```python
from build123d import *

# Parameters (mm, degrees)
SKETCH_1_R          = 21.15
SKETCH_1_R_2        = 1.5
EXTRUDE_1_DEPTH     = 4
SKETCH_2_W          = 6
SKETCH_2_H          = 5
CUT_EXTRUDE_1_DEPTH = 98.49871794


with BuildPart() as part:
    # 草图1 → 凸台-拉伸1 (new body)
    with BuildSketch(Plane.XY):
        with BuildLine():
            Line((-29, 6), (29, 6))
            Line((29, 6), (29, -64))
            ThreePointArc((29, -64), (0, -93), (-29, -64))
            Line((-29, -64), (-29, 6))
        make_face()
        with Locations((0, -64)):
            Circle(SKETCH_1_R, mode=Mode.SUBTRACT)
        with Locations((-17.5, 3)):
            Circle(SKETCH_1_R_2, mode=Mode.SUBTRACT)
        with Locations((17.5, 3)):
            Circle(SKETCH_1_R_2, mode=Mode.SUBTRACT)
        with Locations((18.561553006, -82.561553006)):
            Circle(SKETCH_1_R_2, mode=Mode.SUBTRACT)
        with Locations((-18.561553006, -82.561553006)):
            Circle(SKETCH_1_R_2, mode=Mode.SUBTRACT)
        with Locations((-18.561553006, -45.438446994)):
            Circle(SKETCH_1_R_2, mode=Mode.SUBTRACT)
        with Locations((18.561553006, -45.438446994)):
            Circle(SKETCH_1_R_2, mode=Mode.SUBTRACT)
        with Locations((-17.5, -3)):
            Circle(SKETCH_1_R_2, mode=Mode.SUBTRACT)
        with Locations((17.5, -3)):
            Circle(SKETCH_1_R_2, mode=Mode.SUBTRACT)
    extrude(amount=EXTRUDE_1_DEPTH)

    # 草图2 → 切除-拉伸1 (cut, through all)
    with BuildSketch(Plane.XY.offset(4)):
        with Locations((0, 3.5)):
            Rectangle(SKETCH_2_W, SKETCH_2_H)
    extrude(amount=-CUT_EXTRUDE_1_DEPTH, mode=Mode.SUBTRACT)


solid = part.part
```
Geometry: final body of the model. Coordinates: model frame, mm. A direction names the side the tool comes from. Round coordinates to 2 decimals unless told otherwise and drop trailing zeros. Write each loop counter-clockwise with the first axis right and the second up, starting at its lowest first coordinate (ties: lowest second). Pieces come first, ordered by that corner, then holes. Notation, with made-up numbers: M 24.5,39 L 33.5,39 A19 ccw 33.5,51 Z; hole C -9.75,35.5 d10. An arc over 180 degrees is marked long. Answer in a Markdown table with one row per item. Add a question column.
(1) Contact query for flat-ended pins moving along their axis: pin 1 (3.5 mm diameter, centred on x = -17.5, y = 3, fed in from +Z); pin 2 (2.5 mm diameter, centred on x = -18.56, y = -82.56, fed in from +Z). Output: stop coordinate, or through.
(2) Reachability of faces 5 (the face through (16, 3, 2)), 6 (the face through (-3, 3, 2)) from +Z, -Z, +X, -X, +Y, -Y: full face, straight path, thin tool, end or side. Return the list, or none.
(3) Ray query, L1, parallel to Y at x = -17.5, z = 0.9; L2, parallel to Y at x = 17, z = 2.2; L3, parallel to X at y = -83.5, z = 1.5. Return the intervals inside material, ascending.
(4) Cut plane C-C, the plane z = 1.9. Give the number of separate pieces and of enclosed holes in the cut face, then the cut area to 3 significant figures.
(5) Draft query along Y for faces 1 (the face through (-16, 6, 2)), 2 (the face through (-18.76, -43.95, 1.97)), 3 (the face through (0.638, -92.993, 1.972)), 4 (the face through (3, 3, 2)). Return one class per face: pulls with the +Y half, pulls with the -Y half, needs draft (parallel to the pull), parting line crosses it, or undercut.
(6) Cut plane A-A, the plane y = 3. Return the cut outline in (x, z), then the cut area to 3 significant figures.
(7) Cut plane D-D, the plane y = -77.5. Return the cut outline in (x, z).
(8) Cut plane B-B, the plane x = 0. Return the cut outline in (y, z).
Established:
| question | item | result |
|---|---|---|
| 1 | pin 1 | z = 4 |
| 1 | pin 2 | through |
| 2 | face 5 | +Z, -Z |
| 2 | face 6 | +Z, -Z, +Y |
| 3 | L1 | -87.12 to -83.62, -81.5 to -75.88, -52.12 to -46.5, -44.38 to -4.5, -1.5 to 1.5, 4.5 to 6 |
| 3 | L2 | -87.49 to -76.58, -51.42 to -4.41, -1.59 to 1.59, 4.41 to 6 |
| 3 | L3 | -21.47 to -19.73, -17.39 to -8.19, 8.19 to 17.39, 19.73 to 21.47 |
| 4 | separate pieces | 1 |
| 4 | enclosed holes | 9 |
| 4 | area | 3,890 mm² |
| 5 | face 1 | pulls with the +Y half |
| 5 | face 2 | undercut |
| 5 | face 3 | pulls with the -Y half |
| 5 | face 4 | needs draft |
| 6 | outline | M -29,0 L -19,0 L -19,4 L -29,4 Z; M -16,0 L -3,0 L -3,4 L -16,4 Z; M 3,0 L 16,0 L 16,4 L 3,4 Z; M 19,0 L 29,0 L 29,4 L 19,4 Z |
| 6 | area | 184 mm² |
| 7 | outline | M -25.67,0 L -16.28,0 L -16.28,4 L -25.67,4 Z; M 16.28,0 L 25.67,0 L 25.67,4 L 16.28,4 Z |
| 8 | outline | M -93,0 L -85.15,0 L -85.15,4 L -93,4 Z; M -42.85,0 L 1,0 L 1,4 L -42.85,4 Z |
